Geometry: final body of the model. Coordinates: model frame, mm. Face numbers are marked on the shaded views. A direction names the side the tool comes from. Coordinates: 2 decimals unless noted, no trailing zeros. Loops run counter-clockwise (first coordinate to the right, second up) from the corner with the lowest first, then second, coordinate; pieces in that order, holes last. Notation, with made-up numbers: (58, 28.5) -> (110, 28.5) arc R18 cw to (110, 35.5) -> close; hole circle Ø2 at (35, 81). An arc over 180 degrees is marked (long way). One line per item, written item: value. Start each with the question number.
Item 1: Section query D-D on y = 18.5. Return loops of the section in (x, z) (1 decimal).
Item 2: Section query C-C on z = 30. Return loops of the section in (x, y).
Item 3: Section query B-B on x = -6. Return loops of the section in (y, z).
Item 4: Set-up query: the marked faces 4 and 5. Return all of +Z, -Z, +X, -X, +Y, -Y with unobstructed straight access to the full face (end or side cutting, diameter ignored); none if empty.
Item 5: Mould query, pull axis X, two halves, no side actions, for the marked faces 1, 2 and 3. Classes: +X half, -X half, draft (parallel to the pull), parting line (faces both ways), or undercut.
Item 6: Section query A-A on y = 10.25. Return loops of the section in (x, z).
Item 7: Contact query for flat-ended pins moving along their axis: pin 1 Ø1 at (x, z) = (-1, 15.5) entering from -Y; pin 2 Ø2 at (y, z) = (22, -19.5) entering from +X. Output: stop coordinate, or through.
Item 8: Ray query, probe 1 along Z at (x, y) = (44, 0.9); probe 2 along Z at (x, y) = (-29.5, 8.75); probe 3 along Z at (x, y) = (49.5, 2.05). Return the intervals inside material, ascending. Write a range as from..to.
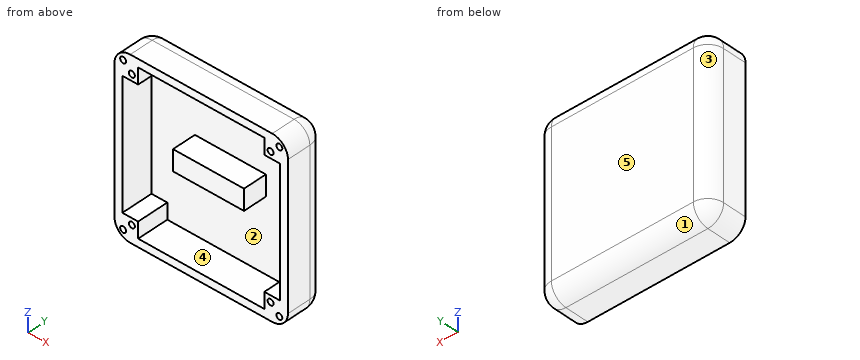
from build123d import *

# Parameters (mm, degrees)
F0_W      = 110
F0_H      = 110
F1_DEPTH  = 25
F2_R      = 10
F3_W      = 110
F3_H      = 110
F4_DEPTH  = 26
F6_DEPTH  = 20
F7_W      = 45
F7_H      = 13
F7_W_2    = 41
F7_H_2    = 9
F8_DEPTH  = 15
F9_W      = 45
F9_H      = 13
F10_DEPTH = 2
F11_R     = 1.9
F12_DEPTH = 3


with BuildPart() as f1:
    # F0 (on Front) → F1 (new body, symmetric)
    with BuildSketch(Plane.XZ):
        Rectangle(F0_W, F0_H)
    extrude(amount=F1_DEPTH, both=True)

    # F2
    f2_edges = [f1.edges().sort_by_distance(p)[0] for p in [
        (0, -25, 55),
        (-55, -25, 0),
        (0, -25, -55),
        (55, -25, 0),
        (55, 25, 0),
        (55, 0, 55),
        (55, 0, -55),
        (0, 25, 55),
        (-55, 0, 55),
        (-55, 25, 0),
        (-55, 0, -55),
        (0, 25, -55),
    ]]
    fillet(f2_edges, radius=F2_R)

    # F3 (on Front) → F4 (cut)
    with BuildSketch(Plane.XZ):
        Rectangle(F3_W, F3_H)
    extrude(amount=F4_DEPTH, mode=Mode.SUBTRACT)

    # F5 (on Front) → F6 (cut)
    with BuildSketch(Plane.XZ):
        Polygon((40, 40), (40, 50), (-40, 50), (-40, 40), (-50, 40), (-50, -40), (-40, -40), (-40, -50), (40, -50), (40, -40), (50, -40), (50, 40), align=None)
    extrude(amount=-F6_DEPTH, mode=Mode.SUBTRACT)

    # F7 (on face) → F8 (join)
    with BuildSketch(Plane.XZ.offset(-20)):
        with Locations((0, 2)):
            Rectangle(F7_W, F7_H)
        with Locations((0, 2)):
            Rectangle(F7_W_2, F7_H_2, mode=Mode.SUBTRACT)
    extrude(amount=F8_DEPTH)

    # F9 (on face) → F10 (join)
    with BuildSketch(Plane.XZ.offset(-5)):
        with Locations((0, 2)):
            Rectangle(F9_W, F9_H)
    extrude(amount=-F10_DEPTH)

    # F11 (on face) → F12 (cut)
    with BuildSketch(Plane.XZ):
        with Locations((49.5, 49.5)):
            Circle(F11_R)
        with Locations((44, 44)):
            Circle(F11_R)
        with Locations((-44, 44)):
            Circle(F11_R)
        with Locations((-49.5, 49.5)):
            Circle(F11_R)
        with Locations((-44, -44)):
            Circle(F11_R)
        with Locations((-49.5, -49.5)):
            Circle(F11_R)
        with Locations((44, -44)):
            Circle(F11_R)
        with Locations((49.5, -49.5)):
            Circle(F11_R)
    extrude(amount=-F12_DEPTH, mode=Mode.SUBTRACT)


solid = f1.part
Reply:
1. outline: (-54.4, -45) arc R9.4 ccw to (-45, -54.4) -> (45, -54.4) arc R9.4 ccw to (54.4, -45) -> (54.4, 45) arc R9.4 ccw to (45, 54.4) -> (-45, 54.4) arc R9.4 ccw to (-54.4, 45) -> close; (-22.5, -4.5) -> (22.5, -4.5) -> (22.5, 8.5) -> (-22.5, 8.5) -> close; hole (-50, -40) -> (-40, -40) -> (-40, -50) -> (40, -50) -> (40, -40) -> (50, -40) -> (50, 40) -> (40, 40) -> (40, 50) -> (-40, 50) -> (-40, 40) -> (-50, 40) -> close; hole (-20.5, -2.5) -> (20.5, -2.5) -> (20.5, 6.5) -> (-20.5, 6.5) -> close
2. outline: (-55, 0) -> (-50, 0) -> (-50, 20) -> (50, 20) -> (50, 0) -> (55, 0) -> (55, 15) arc R10 ccw to (45, 25) -> (-45, 25) arc R10 ccw to (-55, 15) -> close
3. outline: (0, -55) -> (15, -55) arc R10 ccw to (25, -45) -> (25, 45) arc R10 ccw to (15, 55) -> (0, 55) -> (0, 50) -> (20, 50) -> (20, 8.5) -> (5, 8.5) -> (5, -4.5) -> (20, -4.5) -> (20, -50) -> (0, -50) -> close; hole (7, -2.5) -> (20, -2.5) -> (20, 6.5) -> (7, 6.5) -> close
4. face 4: -Y
4. face 5: +Z, -Z, +X, -X, +Y
5. face 1: draft
5. face 2: undercut
5. face 3: -X half
6. outline: (-55, -45) arc R10 ccw to (-45, -55) -> (45, -55) arc R10 ccw to (55, -45) -> (55, 45) arc R10 ccw to (45, 55) -> (-45, 55) arc R10 ccw to (-55, 45) -> close; (-22.5, -4.5) -> (22.5, -4.5) -> (22.5, 8.5) -> (-22.5, 8.5) -> close; hole (-50, -40) -> (-40, -40) -> (-40, -50) -> (40, -50) -> (40, -40) -> (50, -40) -> (50, 40) -> (40, 40) -> (40, 50) -> (-40, 50) -> (-40, 40) -> (-50, 40) -> close; hole (-20.5, -2.5) -> (20.5, -2.5) -> (20.5, 6.5) -> (-20.5, 6.5) -> close
7. pin 1: stops at y = 20
7. pin 2: stops at x = 53
8. probe 1: z = -55..-45.9, -42.1..-40, 40..42.1, 45.9..55
8. probe 2: z = -55..-50, 50..55
8. probe 3: z = -53.93..-51.4, -47.6..-40, 40..47.6, 51.4..53.93
